```python
from build123d import *

# Parameters (mm, degrees)
F0_W     = 1
F0_H     = 2.4
F1_DEPTH = 15


# Not quite as in the source:
# - a feature names something its author has since deleted; it is built from what else it names


with BuildPart() as f1:
    # F0 (on Top) → F1 (new body)
    with BuildSketch(Plane.XY):
        with Locations((10.8, -6.7)):
            Rectangle(F0_W, F0_H)
        with Locations((-10.8, -6.7)):
            Rectangle(F0_W, F0_H)
        Polygon((-2.45, -8.5), (-2.45, -7.9), (-3.85, -7.9), (-1.45, -10.5), (-1.45, -8.5), align=None)
        with BuildLine():
            Line((10.3, -4.5), (10.3, -5.5))
            Line((10.3, -5.5), (11.3, -5.5))
            ThreePointArc((11.3, -5.5), (11.0071067812, -4.7928932188), (10.3, -4.5))
        make_face()
        Polygon((-1.45, -5.5), (-2.45, -5.5), (-2.45, -7.9), (-2.45, -8.5), (-1.45, -8.5), align=None)
        Polygon((2.45, -5.5), (1.45, -5.5), (1.45, -8.5), (2.45, -8.5), (2.45, -7.9), align=None)
        with BuildLine():
            Line((-11.3, -5.5), (-10.3, -5.5))
            Line((-10.3, -5.5), (-2.45, -5.5))
            Line((-2.45, -5.5), (-1.45, -5.5))
            Line((-1.45, -5.5), (1.45, -5.5))
            Line((1.45, -5.5), (2.45, -5.5))
            Line((2.45, -5.5), (10.3, -5.5))
            Line((10.3, -5.5), (10.3, -4.5))
            Line((10.3, -4.5), (6.9, -4.5))
            ThreePointArc((6.9, -4.5), (-1.5852813742, -0.9852813742), (-5.1, 7.5))
            Line((-5.1, 7.5), (-5.1, 9))
            ThreePointArc((-5.1, 9), (-5.5393398282, 10.0606601718), (-6.6, 10.5))
            Line((-6.6, 10.5), (-7.1, 10.5))
            Line((-7.1, 10.5), (-7.1, -4))
            Line((-7.1, -4), (-9.3, -4))
            Line((-9.3, -4), (-9.3, 10.5))
            Line((-9.3, 10.5), (-9.8, 10.5))
            ThreePointArc((-9.8, 10.5), (-10.8606601718, 10.0606601718), (-11.3, 9))
            Line((-11.3, 9), (-11.3, -5.5))
        make_face()
        Polygon((2.45, -8.5), (1.45, -8.5), (1.45, -10.5), (3.85, -7.9), (2.45, -7.9), align=None)
    extrude(amount=F1_DEPTH)


solid = f1.part
```
Could you check a few things on this model? Use its own coordinates, in mm. A direction names the side the tool comes from. Round coordinates to 2 decimals unless told otherwise and drop trailing zeros. Loops run counter-clockwise (first coordinate to the right, second up) from the corner with the lowest first, then second, coordinate; pieces in that order, holes last. Notation, with made-up numbers: M 51.25,81.5 L 58.25,81.5 A20 ccw 58.25,116.5 Z; hole C 53,66 d6. An arc over 180 degrees is marked long. Put each result on its own line as item: value.
Q1. I need wall thicknesses on probe 1 along X at (y, z) = (-6.5, 7); probe 2 along Y at (x, z) = (-3, 3.25); probe 3 along X at (y, z) = (9.5, 7). Which ranges of each line are inside material? Lowest first, please.
Check result:
probe 1: -11.3 to -10.3, -2.45 to -1.45, 1.45 to 2.45, 10.3 to 11.3
probe 2: -8.82 to -7.9, -5.5 to 0.72
probe 3: -11.21 to -9.3, -7.1 to -5.19
Q2. Imagine slicing it at C-C (x = -3). Write out the boundary of the cut face in (y, z).
Check result:
outline: M -8.82,0 L -7.9,0 L -7.9,15 L -8.82,15 Z; M -5.5,0 L 0.72,0 L 0.72,15 L -5.5,15 Z
Q3. Imagine slicing it at B-B (y = 8). Write out the boundary of the cut face in (x, z), then the cut area to 3 significant figures.
Check result:
outline: M -11.3,0 L -9.3,0 L -9.3,15 L -11.3,15 Z; M -7.1,0 L -5.1,0 L -5.1,15 L -7.1,15 Z
area: 60.0 mm2
Q4. Imagine slicing it at A-A (y = -7). Write out the boundary of the cut face in (x, z).
Check result:
outline: M -11.3,0 L -10.3,0 L -10.3,15 L -11.3,15 Z; M -2.45,0 L -1.45,0 L -1.45,15 L -2.45,15 Z; M 1.45,0 L 2.45,0 L 2.45,15 L 1.45,15 Z; M 10.3,0 L 11.3,0 L 11.3,15 L 10.3,15 Z
Q5. For pin 1 (1.5 mm diameter, centred on x = 6.5, z = 7, fed in from -Y); pin 2 (1 mm diameter, centred on x = 9, z = 7, fed in from +Y); pin 3 (4 mm diameter, centred on x = 7, z = 8.5, fed in from +Y); pin 4 (8 mm diameter, centred on x = 5.5, y = 3.5, fed in from +Z), each with a flat end and sliding along its axis, tell me the tip position at first contact or that it passes through.
Check result:
pin 1: y = -5.5
pin 2: y = -4.5
pin 3: y = -4.35
pin 4: through
Q6. Thinking about a two-plate mould opening in X: for faces 5 (the face through (-4, -1, 15)), 6 (the face through (-5.1, 8, 7)), 7 (the face through (-9.3, 3, 7)), which applies, released by +X, released by -X, zero draft, split by the parting line, or undercut?
Check result:
face 5: zero draft
face 6: released by +X
face 7: undercut
Q7. Imagine slicing it at D-D (z = 7.75). Write out the boundary of the cut face in (x, y), then the cut area to 3 significant figures.
Check result:
outline: M -11.3,-7.9 L -10.3,-7.9 L -10.3,-5.5 L -2.45,-5.5 L -2.45,-7.9 L -3.85,-7.9 L -1.45,-10.5 L -1.45,-5.5 L 1.45,-5.5 L 1.45,-10.5 L 3.85,-7.9 L 2.45,-7.9 L 2.45,-5.5 L 10.3,-5.5 L 10.3,-7.9 L 11.3,-7.9 L 11.3,-5.5 A1 ccw 10.3,-4.5 L 6.9,-4.5 A12 cw -5.1,7.5 L -5.1,9 A1.5 ccw -6.6,10.5 L -7.1,10.5 L -7.1,-4 L -9.3,-4 L -9.3,10.5 L -9.8,10.5 A1.5 ccw -11.3,9 Z
area: 129 mm2
Q8. On a 3-axis mill with a long thin cutter (end or side, diameter ignored), from which of +Z, -Z, +X, -X, +Y, -Y can I reach the whole of each face in a straight line? I mean faces 1 (the face through (-7.1, 3, 7)), 2 (the face through (6, -5.5, 7)), 3 (the face through (0, -5.5, 7)), 4 (the face through (11, -7.9, 7)). Say none if no direction works.
Check result:
face 1: +Z, -Z, +Y
face 2: +Z, -Z
face 3: +Z, -Z, -Y
face 4: +Z, -Z, +X, -Y
